Source: CAD feature listing. Evaluate the final solid. Frame: model axes, mm. A direction names the side the tool comes from. Coordinates: 2 decimals unless noted, no trailing zeros. Order: outer loops, then holes, each group sorted by start corner. A loop starts at its lowest first (then second) coordinate and runs counter-clockwise, first axis right, second up.
```python
from build123d import *

# Parameters (mm, degrees)
SKETCH1_W           = 40
SKETCH1_H           = 30
BOSS_EXTRUDE1_DEPTH = 5
SKETCH2_W           = 5
SKETCH2_H           = 30
BOSS_EXTRUDE2_DEPTH = 35
BOSS_EXTRUDE3_DEPTH = 5
BOSS_EXTRUDE4_DEPTH = 5
CUT_EXTRUDE1_DEPTH  = 5
CUT_EXTRUDE2_DEPTH  = 5
FILLET4_R           = 12
FILLET5_R           = 12
FILLET6_R           = 5


with BuildPart() as part:
    # Sketch1 → Boss-Extrude1 (new body)
    with BuildSketch(Plane(origin=(0, 0, 0), x_dir=(1, 0, 0), z_dir=(0, 1, 0))):
        with Locations((20, 15)):
            Rectangle(SKETCH1_W, SKETCH1_H)
    extrude(amount=BOSS_EXTRUDE1_DEPTH)

    # Sketch2 → Boss-Extrude2 (add)
    with BuildSketch(Plane(origin=(0, 5, 0), x_dir=(1, 0, 0), z_dir=(0, 1, 0))):
        with Locations((2.5, 15)):
            Rectangle(SKETCH2_W, SKETCH2_H)
    extrude(amount=BOSS_EXTRUDE2_DEPTH)

    # Sketch3 → Boss-Extrude3 (add)
    with BuildSketch(Plane.XY):
        Polygon((5, 40), (40, 5), (5, 5), align=None)
    extrude(amount=-BOSS_EXTRUDE3_DEPTH)

    # Sketch4 → Boss-Extrude4 (add)
    with BuildSketch(Plane(origin=(0, 0, -30), x_dir=(-1, 0, 0), z_dir=(0, 0, -1))):
        Polygon((-40, 5), (-5, 40), (-5, 5), align=None)
    extrude(amount=-BOSS_EXTRUDE4_DEPTH)

    # Sketch5 → Cut-Extrude1 (cut)
    with BuildSketch(Plane.XZ):
        with BuildLine():
            Line((15, -12.5), (25, -12.5))
            ThreePointArc((25, -12.5), (27.5, -15), (25, -17.5))
            Line((25, -17.5), (15, -17.5))
            ThreePointArc((15, -17.5), (12.5, -15), (15, -12.5))
        make_face()
    extrude(amount=-CUT_EXTRUDE1_DEPTH, mode=Mode.SUBTRACT)

    # Sketch6 → Cut-Extrude2 (cut)
    with BuildSketch(Plane.ZY):
        with BuildLine():
            Line((-12.5, 25), (-12.5, 15))
            ThreePointArc((-12.5, 15), (-15, 12.5), (-17.5, 15))
            Line((-17.5, 15), (-17.5, 25))
            ThreePointArc((-17.5, 25), (-15, 27.5), (-12.5, 25))
        make_face()
    extrude(amount=-CUT_EXTRUDE2_DEPTH, mode=Mode.SUBTRACT)

    # Fillet4
    # the kernel refuses this fillet: 12 mm, written as the material it takes off along each edge
    with BuildSketch(Plane(origin=(40, 5, 12.426406871), x_dir=(-0.7071067811865481, 0.707106781186547, 0), z_dir=(0, 0, -1))) as fillet4_piece_1:
        with BuildLine():
            CenterArc((FILLET4_R * 0.414213562373, -FILLET4_R), FILLET4_R, 90, 45)
            Line((-FILLET4_R * 0.292893218813, -FILLET4_R * 0.292893218813), (0, 0))
            Line((0, 0), (FILLET4_R * 0.414213562373, 0))
        make_face()
    extrude(amount=29.852813742, mode=Mode.SUBTRACT)
    with BuildSketch(Plane(origin=(40, 5, -12.573593129), x_dir=(0, -1, 0), z_dir=(0, 0, -1))) as fillet4_piece_2:
        with BuildLine():
            CenterArc((FILLET4_R * 0.414213562373, FILLET4_R), FILLET4_R, 225, 45)
            Line((-FILLET4_R * 0.292893218813, FILLET4_R * 0.292893218813), (0, 0))
            Line((0, 0), (FILLET4_R * 0.414213562373, 0))
        make_face()
    extrude(amount=29.852813742, mode=Mode.SUBTRACT)

    # Fillet5
    # the kernel refuses this fillet: 12 mm, written as the material it takes off along each edge
    with BuildSketch(Plane(origin=(5, 40, -17.426406871), x_dir=(-1, 0, 0), z_dir=(0, 0, 1)), Plane(origin=(5, 40, -42.426406871), x_dir=(-1, 0, 0), z_dir=(0, 0, 1))) as fillet5_piece_1:
        with BuildLine():
            CenterArc((FILLET5_R * 0.414213562373, FILLET5_R), FILLET5_R, 225, 45)
            Line((-FILLET5_R * 0.292893218813, FILLET5_R * 0.292893218813), (0, 0))
            Line((0, 0), (FILLET5_R * 0.414213562373, 0))
        make_face()
    extrude(amount=29.852813742, mode=Mode.SUBTRACT)

    # Fillet6
    fillet6_edges = [part.edges().sort_by_distance(p)[0] for p in [
        (0, 0, -15),
    ]]
    fillet(fillet6_edges, radius=FILLET6_R)


solid = part.part
```
1. Section query D-D on y = 30.5. Return loops of the section in (x, z).
Findings:
outline: (0, -30) - (14.5, -30) - (14.5, -25) - (5, -25) - (5, -5) - (14.5, -5) - (14.5, 0) - (0, 0) - close
2. Access query for faces 1 (the face through (22, 5, -11)), 2 (the face through (2, 20, -17.5)), 3 (the face through (27.5, 2.5, -14.9)). Directions: +Z, -Z, +X, -X, +Y, -Y. A direction counts if a zero-diameter tool reaches every point of the face in a straight line with its end or side. Return the directions, or none.
Findings:
face 1: +X, +Y
face 2: +X, -X
face 3: +Y, -Y
3. Pin query (flat end, axial travel): P1, Ø4, axis at y = 8, z = -8.5, coming from the +X side; P2, Ø1, axis at x = 13, z = -4.5, coming from the +Y side; P3, Ø10, axis at x = 20, z = -16, coming from the +Y side; P4, Ø6, axis at x = 18, y = 29.5, coming from the -Z side. Return the tip coordinate at first contact, or that it passes through.
Findings:
P1: stops at x = 5
P2: stops at y = 32.5
P3: stops at y = 5
P4: stops at z = -30
4. Section query C-C on x = 10.5. Return loops of the section in (y, z).
Findings:
outline: (0, -30) - (34.5, -30) - (34.5, -25) - (5, -25) - (5, -5) - (34.5, -5) - (34.5, 0) - (0, 0) - close
5. Section query A-A on z = -15. Count the separate pieces of the cut face and the enclosed holes in it, plus the area to 3 significant figures.
Findings:
separate pieces: 3
enclosed holes: 0
area: 216 mm2
6. Ray query, line 1 (Z direction, x = 12, y = 11); line 2 (Z direction, x = 2, y = 16); line 3 (X direction, y = 36.5, z = -15.5). Return the intervals inside material, ascending.
Findings:
line 1: z = -30 to -25, -5 to 0
line 2: z = -30 to -17.5, -12.5 to 0
line 3: x = 0 to 5
7. Draft query along Z for faces 4 (the face through (5, 22, -19)), 5 (the face through (22, 0, -19)), 6 (the face through (20, 2, -17.5)), 7 (the face through (15, 16, -30)). Return one class per face: released by +Z, released by -Z, zero draft, split by the parting line, or undercut.
Findings:
face 4: undercut
face 5: zero draft
face 6: undercut
face 7: released by -Z
8. Section query B-B on y = 19. Return loops of the section in (x, z), plus the area to 3 significant figures.
Findings:
outline: (0, -30) - (26, -30) - (26, -25) - (5, -25) - (5, -17.5) - (0, -17.5) - close; (0, -12.5) - (5, -12.5) - (5, -5) - (26, -5) - (26, 0) - (0, 0) - close
area: 335 mm2
